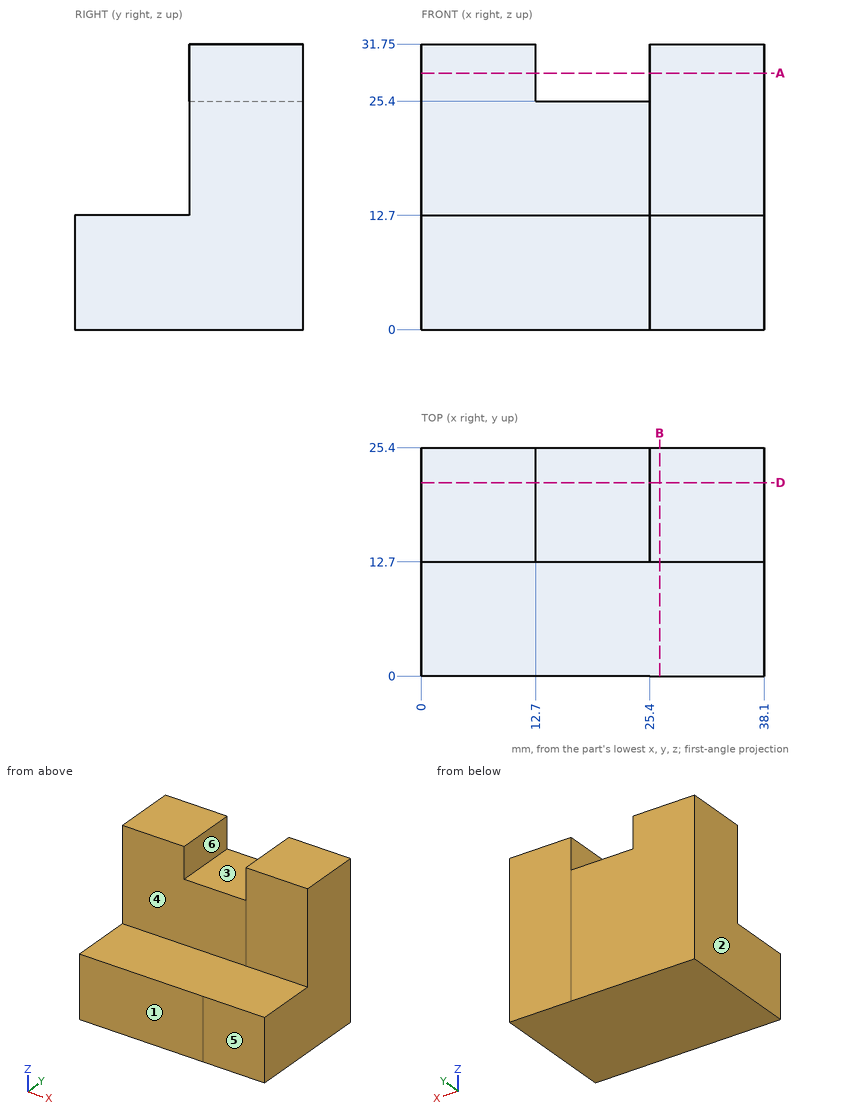
Here's the drawing with two shaded views (mm, measured from the low corner). I have some questions. A direction names the side the tool comes from. Give positions to 0.01 mm unless a question says otherwise; leave off trailing zeros. Loops run counter-clockwise (first coordinate to the right, second up) from the corner with the lowest first, then second, coordinate; pieces in that order, holes last. Notation, with made-up numbers: M 37,-16.5 L 82,-16.5 A30 ccw 82,12.5 Z; hole C -37.75,82 d1. An arc over 180 degrees is marked long. One line per item, written item: value. Start each with the question number.
1) I'm going to push flat-ended pins straight in: pin 1 (4 mm diameter, centred on x = 27, y = 5.5, fed in from +Z); pin 2 (6.5 mm diameter, centred on x = 19.5, y = 21.5, fed in from +Z); pin 3 (6.5 mm diameter, centred on x = 29.5, z = 26.5, fed in from -Y). Where does each tip first touch, or does it pass through?
2) If we section it at D-D, the plane y = 21.5: Write out the boundary of the cut face in (x, z), and give its area (3 significant figures).
3) On a 3-axis mill with a long thin cutter (end or side, diameter ignored), from which of +Z, -Z, +X, -X, +Y, -Y can I reach the whole of each face in a straight line? I mean the marked faces 4, 5 and 6. Say none if no direction works.
4) If we section it at A-A, the plane z = 28.5: Write out the boundary of the cut face in (x, y).
5) If we section it at B-B, the plane x = 26.5: Write out the boundary of the cut face in (y, z), and give its area (3 significant figures).
6) Thinking about a two-plate mould opening in X: for the marked faces 1, 2 and 3, which applies, +X half, -X half, draft (parallel to the pull), parting line (faces both ways), or undercut?
7) If I drill on line 1 (Y direction, x = 33.5, z = 14); line 2 (Z direction, x = 18, y = 1.25); line 3 (Z direction, x = 18, y = 12.75), over which ranges is the centre line in solid material (lowest first)? Write a range as [from, to].
Completed:
1. pin 1: stops at z = 12.7
1. pin 2: stops at z = 25.4
1. pin 3: stops at y = 12.7
2. outline: M 0,0 L 38.1,0 L 38.1,31.75 L 25.4,31.75 L 25.4,25.4 L 12.7,25.4 L 12.7,31.75 L 0,31.75 Z
2. area: 1,130 mm^2
3. face 4: +Z, +X, -X, -Y
3. face 5: +Z, -Z, +X, -X, -Y
3. face 6: +Z, +Y, -Y
4. outline: M 0,12.7 L 12.7,12.7 L 12.7,25.4 L 0,25.4 Z; M 25.4,12.7 L 38.1,12.7 L 38.1,25.4 L 25.4,25.4 Z
5. outline: M 0,0 L 25.4,0 L 25.4,31.75 L 12.7,31.75 L 12.7,12.7 L 0,12.7 Z
5. area: 565 mm^2
6. face 1: draft
6. face 2: -X half
6. face 3: undercut
7. line 1: y = [12.7, 25.4]
7. line 2: z = [0, 12.7]
7. line 3: z = [0, 25.4]
